Autodesk Inventor part; units mm, degrees
ref_plane "YZ Plane" through (0, 0, 0) normal (1, 0, 0) x (0, 1, 0)
ref_plane "XZ Plane" through (0, 0, 0) normal (0, 1, 0) x (-1, 0, 0)
ref_plane "XY Plane" through (0, 0, 0) normal (0, 0, 1) x (1, 0, 0)
sketch "Náčrt1" plane through (0, 0, 0) normal (0, 0, 1) x (1, 0, 0)
  line L0 (-6, -5) -> (6, -5)
  line L1 (6, -5) -> (6, 5)
  line L2 (6, 5) -> (-6, 5)
  line L3 (-6, 5) -> (-6, -5)
  point P0 (0, 0)
  dimension "d2" = 12
  dimension "d3" = 10
  dimension "d4" = 6
  dimension "d5" = 5
extrude "Vysunutí1" add sketch "Náčrt1" along normal blind 25
sketch "Náčrt2" plane through (0, 0, 25) normal (0, 0, 1) x (1, 0, 0)
  circle A0 centre (0, 0) radius 1.5
  dimension "d8" = 3
extrude "Vysunutí2" add sketch "Náčrt2" along normal blind 10
properties part number "motor GA12-N20 12V s převodovkou"
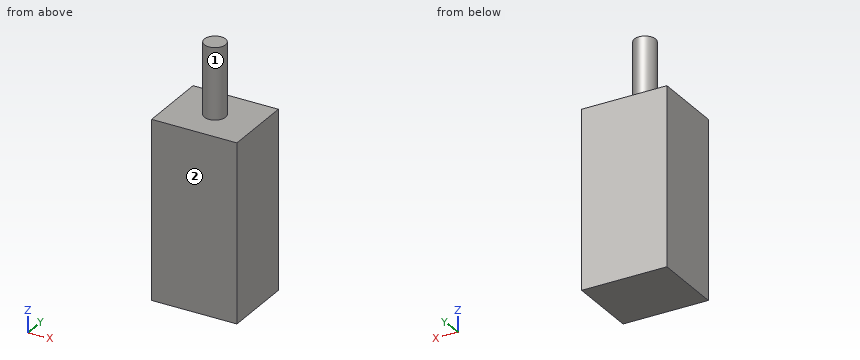
The model under review builds one solid part; all positions refer to its coordinate system, in mm. Face numbers are marked on the shaded views. A direction names the side the tool comes from. Coordinates: 2 decimals unless noted, no trailing zeros. Write each loop counter-clockwise with the first axis right and the second up, starting at its lowest first coordinate (ties: lowest second). Pieces come first, ordered by that corner, then holes. Notation, with made-up numbers: (26, 38) - (45, 38) arc R11 ccw to (45, 59) - close; hole circle Ø1 at (-37, 33.5). An arc over 180 degrees is marked (long way). Answer as CSV lines item,"result".
(1) We need section A-A (y = 0). Give the boundary of the cut face in (x, z).
Data:
outline,"(-6, 0) - (6, 0) - (6, 25) - (1.5, 25) - (1.5, 35) - (-1.5, 35) - (-1.5, 25) - (-6, 25) - close"
(2) We need section B-B (x = 0). Give the boundary of the cut face in (y, z), plus the area to 3 significant figures.
Data:
outline,"(-5, 0) - (5, 0) - (5, 25) - (1.5, 25) - (1.5, 35) - (-1.5, 35) - (-1.5, 25) - (-5, 25) - close"
area,"280 mm2"
(3) Tool access review of the marked faces 1 and 2: name each direction out of +Z, -Z, +X, -X, +Y, -Y from which nothing blocks a thin tool from reaching the whole face with its end or side.
Data:
face 1,"+Z"
face 2,"+Z, -Z, +X, -X, -Y"
(4) We need section C-C (y = 3.25). Give the boundary of the cut face in (x, z), plus the area to 3 significant figures.
Data:
outline,"(-6, 0) - (6, 0) - (6, 25) - (-6, 25) - close"
area,"300 mm2"
(5) We need section D-D (x = -2). Give the boundary of the cut face in (y, z).
Data:
outline,"(-5, 0) - (5, 0) - (5, 25) - (-5, 25) - close"
(6) For line 1 along Z through (x, y) = (3.5, 4.75); line 2 along X through (y, z) = (0.75, 26); line 3 along X through (y, z) = (1, 28.5), list the stretches that pass through material, from the lowest coordinate up. Write a range as [from, to].
Data:
line 1,"z = [0, 25]"
line 2,"x = [-1.3, 1.3]"
line 3,"x = [-1.12, 1.12]"
